Part print with two shaded views. Sizes in mm from the minimum x, y, z corner. A direction names the side the tool comes from. Round coordinates to 2 decimals unless told otherwise and drop trailing zeros. Loops run counter-clockwise (first coordinate to the right, second up) from the corner with the lowest first, then second, coordinate; pieces in that order, holes last.
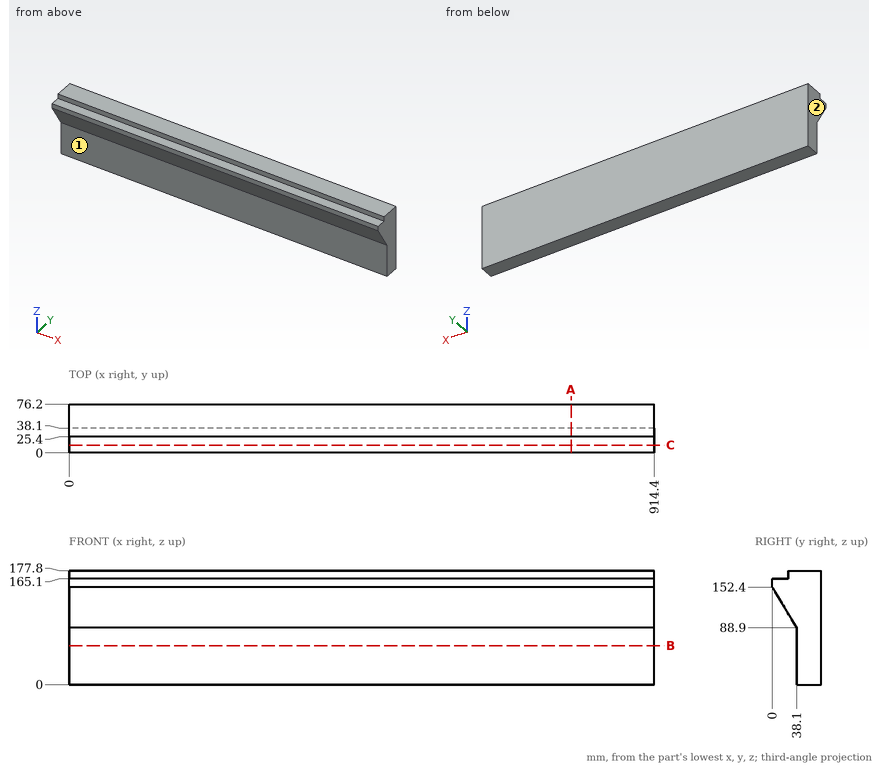
Item 1: Cut at B-B (z = 61). List the corners of the cut face in (x, y).
Verdict:
outline: (0, 38.1) - (914.4, 38.1) - (914.4, 76.2) - (0, 76.2) - close
Item 2: 3-axis set-ups, long thin cutter, end or side, ignore diameter. For the marked faces 1 and 2: which of +Z, -Z, +X, -X, +Y, -Y reach the whole face in a straight line?
Verdict:
face 1: -Z, +X, -X, -Y
face 2: +Z, -Z, -X, +Y, -Y
Item 3: Cut at C-C (y = 12). List the corners of the cut face in (x, z).
Verdict:
outline: (0, 132.4) - (914.4, 132.4) - (914.4, 165.1) - (0, 165.1) - close
Item 4: Wall check: L1, parallel to Y at x = 479, z = 54; L2, parallel to Y at x = 342.5, z = 135; L3, parallel to Z at x = 44.5, y = 21. Give the ranges that are in metal, low to high.
Verdict:
L1: y = 38.1 to 76.2
L2: y = 10.44 to 76.2
L3: z = 117.4 to 165.1
Item 5: Flat gauge pins, fed straight in: P1, Ø20.5, axis at x = 247, y = 11, coming from the +Z side; P2, Ø4, axis at x = 97.5, z = 53.5, coming from the -Y side; P3, Ø10, axis at x = 154.5, z = 142, coming from the -Y side. Where does each tip first touch, or does it go through?
Verdict:
P1: stops at z = 165.1
P2: stops at y = 38.1
P3: stops at y = 3.24
Item 6: Cut at A-A (x = 784.5). List the corners of the cut face in (y, z).
Verdict:
outline: (0, 152.4) - (38.1, 88.9) - (38.1, 0) - (76.2, 0) - (76.2, 177.8) - (25.4, 177.8) - (25.4, 165.1) - (0, 165.1) - close
